from build123d import *

# Parameters (mm, degrees)
SKETCH1_R                    = 10
BOSS_EXTRUDE1_DEPTH          = 15
SKETCH2_R                    = 9
SKETCH2_R_2                  = 4
CUT_EXTRUDE1_DEPTH           = 0.5
M2_5X0_45_TAPPED_HOLE1_D     = 2.05
M2_5X0_45_TAPPED_HOLE1_DEPTH = 6.35
M2_5X0_45_TAPPED_HOLE1_TIP   = 0.615882135


with BuildPart() as part:
    # Sketch1 → Boss-Extrude1 (new body)
    with BuildSketch(Plane(origin=(0, 0, 0), x_dir=(1, 0, 0), z_dir=(0, 1, 0))):
        with Locations(Location((0, 0, 0), (0, 0, 270))):
            Circle(SKETCH1_R)
    extrude(amount=BOSS_EXTRUDE1_DEPTH)

    # Sketch2 → Cut-Extrude1 (cut)
    with BuildSketch(Plane(origin=(0, 15, 0), x_dir=(1, 0, 0), z_dir=(0, 1, 0))):
        with Locations(Location((0, 0, 0), (0, 0, 270))):
            Circle(SKETCH2_R)
        with Locations(Location((0, 0, 0), (0, 0, 270))):
            Circle(SKETCH2_R_2, mode=Mode.SUBTRACT)
    extrude(amount=-CUT_EXTRUDE1_DEPTH, mode=Mode.SUBTRACT)

    # M2.5x0.45 Tapped Hole1
    with Locations(Plane(origin=(0, 0, 0), x_dir=(-1, 0, 0), z_dir=(0, -1, 0))):
        with Locations((0, 0)):
            Hole(M2_5X0_45_TAPPED_HOLE1_D / 2, depth=M2_5X0_45_TAPPED_HOLE1_DEPTH)
            with Locations((0, 0, -(M2_5X0_45_TAPPED_HOLE1_DEPTH + M2_5X0_45_TAPPED_HOLE1_TIP / 2))):  # 118° drill point
                Cone(0, M2_5X0_45_TAPPED_HOLE1_D / 2, M2_5X0_45_TAPPED_HOLE1_TIP, mode=Mode.SUBTRACT)


solid = part.part
Verification items for the finished model (mm, model axes). A direction names the side the tool comes from. Give positions to 0.01 mm unless a question says otherwise; leave off trailing zeros. Loops run counter-clockwise (first coordinate to the right, second up) from the corner with the lowest first, then second, coordinate; pieces in that order, holes last.
1) Sectioned sample at A-A, the plane y = 5.5. Enter the section's corners in (x, z) (3 decimals), then the cut area to 3 significant figures.
2) Sectioned sample at B-B, the plane x = -2.5. Enter the section's corners in (y, z), then the cut area to 3 significant figures.
3) Thickness scan on line 1 along X through (y, z) = (14.85, 0); line 2 along Y through (x, z) = (-6, 4.25); line 3 along X through (y, z) = (9, -0.25). Record the ranges inside material, lowest first.
4) Draft check along Z on faces 1 (the flat face through (0, 15, 0)), 2 (the cylindrical face through (2.703, 14.754, 8.584)), 3 (the cylindrical face through (-9.76, 7.4, -2.17)). Enter one of: pulls with the +Z half, pulls with the -Z half, needs draft (parallel to the pull), parting line crosses it, or undercut.
5) Sectioned sample at D-D, the plane y = 10.75. Enter the section's corners in (x, z).
6) Depth check by flat-ended pin: pin 1 Ø8 at (y, z) = (13, -5) entering from +X; pin 2 Ø1.5 at (x, z) = (4, -3.5) entering from +Y; pin 3 Ø1.5 at (y, z) = (4, -2) entering from -X. Enter the tip coordinate at first touch or a pass-through.
7) Set-up check for faces 4 (the flat face through (0, 0, 2)), 5 (the flat face through (-2, 14.5, 4)), 6 (the cylindrical face through (-0.133, 3.219, -1.016)): record each of +Z, -Z, +X, -X, +Y, -Y from which the full face is reachable in a straight line by a thin tool's end or side.
8) Sectioned sample at C-C, the plane z = -4.5. Enter the section's corners in (x, y), then the cut area to 3 significant figures.
Answers:
1. outline: circle Ø20 at (0, 0); hole circle Ø2.05 at (0, 0)
1. area: 311 mm2
2. outline: (0, -9.68) - (15, -9.68) - (15, -8.65) - (14.5, -8.65) - (14.5, -3.12) - (15, -3.12) - (15, 3.12) - (14.5, 3.12) - (14.5, 8.65) - (15, 8.65) - (15, 9.68) - (0, 9.68) - close
2. area: 285 mm2
3. line 1: x = -10 to -9, -4 to 4, 9 to 10
3. line 2: y = 0 to 14.5
3. line 3: x = -10 to 10
4. face 1: needs draft
4. face 2: undercut
4. face 3: parting line crosses it
5. outline: circle Ø20 at (0, 0)
6. pin 1: stops at x = 9.95
6. pin 2: stops at y = 14.5
6. pin 3: stops at x = -9.92
7. face 4: +Z, -Z, +X, -X, -Y
7. face 5: +Y
7. face 6: -Y
8. outline: (-8.93, 0) - (8.93, 0) - (8.93, 15) - (7.79, 15) - (7.79, 14.5) - (-7.79, 14.5) - (-7.79, 15) - (-8.93, 15) - close
8. area: 260 mm2
